Can you work these out from the model? Positions are in its coordinate system, mm. Face numbers are marked on the shaded views. A direction names the side the tool comes from. Coordinates: 2 decimals unless noted, no trailing zeros. Order: outer loops, then holes, each group sorted by start corner. A loop starts at its lowest first (then second) coordinate and runs counter-clockwise, first axis right, second up. Notation, with made-up numbers: (35, 77.5) - (92, 77.5) arc R22 ccw to (92, 115.5) - close; hole circle Ø2 at (35.5, 21). An arc over 180 degrees is marked (long way). Use a Markdown table: item, result. Add a question column.
(1) I want a section at C-C (z = 1.6). List the corners of the cut face in (x, y) for me, and give its area (3 significant figures).
(2) I want a section at D-D (y = 14). List the corners of the cut face in (x, z) for me, and give its area (3 significant figures).
(3) If I drill on L1, parallel to Y at x = 9.75, z = 1.5; L2, parallel to X at y = 9, z = 0.8; L3, parallel to X at y = 3.5, z = 2.2, over which ranges is the centre line in solid material (lowest first)? Write a range as [from, to].
(4) For pin 1 Ø0.6 at (x, z) = (11.5, 2) entering from -Y; pin 2 Ø0.8 at (x, z) = (12, 0.5) entering from -Y; pin 3 Ø5 at (x, y) = (-1, 13.5) entering from -Z; pin 4 Ø0.6 at (x, y) = (9, 17.5) entering from -Z, each with a flat end and sliding along its axis, tell me the tip position at first contact or that it passes through.
(5) On a 3-axis mill with a long thin cutter (end or side, diameter ignored), from which of +Z, -Z, +X, -X, +Y, -Y can I reach the whole of each face in a straight line? I mean the marked faces 1, 2 and 3. Say none if no direction works.
(6) I want a section at A-A (z = 0.5). List the corners of the cut face in (x, y) for me, and give its area (3 significant figures).
(7) I want a section at B-B (x = 7.5). List the corners of the cut face in (y, z) for me, and give its area (3 significant figures).
```python
from build123d import *

# Parameters (mm, degrees)
F1_DEPTH      = 2.35
F2_R          = 0.5
F3_DEPTH      = 5
F3_DEPTH_BACK = 5
F5_DEPTH      = 1.85
F6_R          = 0.35
F7_DEPTH      = 1.6


with BuildPart() as f1:
    # F0 (on Top) → F1 (new body)
    with BuildSketch(Plane.XY):
        with BuildLine():
            Line((12.5348381698, 18.1987490505), (10.8179235831, 18.1987490505))
            Line((10.8179235831, 18.1987490505), (9.1010301327, 18.1902297699))
            Line((9.1010301327, 18.1902297699), (7.1743787806, 17.653559883))
            Line((7.1743787806, 17.653559883), (3.98264217, 12.5729282876))
            ThreePointArc((3.98264217, 12.5729282876), (3.2243689245, 9.1481475257), (4.0165917388, 5.7310603752))
            Line((4.0165917388, 5.7310603752), (7.2585904547, 0.6823531817))
            Line((7.2585904547, 0.6823531817), (9.1909860265, 0.0613885547))
            Line((9.1909860265, 0.0613885547), (10.8629018068, 0.0696846546))
            Line((10.8629018068, 0.0696846546), (12.5348381698, 0.0696846546))
            Line((12.5348381698, 0.0696846546), (14.464128744, 0.7002301281))
            Line((14.464128744, 0.7002301281), (17.6810360095, 5.7649618728))
            ThreePointArc((17.6810360095, 5.7649618728), (18.4562935833, 9.1859379434), (17.6810360095, 12.606914014))
            Line((17.6810360095, 12.606914014), (14.464128744, 17.6716457586))
            Line((14.464128744, 17.6716457586), (12.5348381698, 18.1987490505))
        make_face()
    extrude(amount=F1_DEPTH)

    # F2 (on Right) → F3 (join, two sides)
    with BuildSketch(Plane.YZ) as f3_sk:
        with Locations((9.1614143501, 1.6)):
            Circle(F2_R)
    extrude(amount=F3_DEPTH)
    extrude(f3_sk.sketch, amount=-F3_DEPTH_BACK)

    # F4 (on face) → F5 (cut)
    with BuildSketch(Plane(origin=(0, 0, 0), x_dir=(1, 0, 0), z_dir=(0, 0, -1))):
        Polygon((7.2585904547, -0.6823531817), (7.0886202668, -0.9470447456), (9.2218469568, -0.2615441498), (10.8624056067, -0.2696846546), (12.5029844531, -0.2696846546), (14.6327834476, -0.9657618207), (14.464128744, -0.7002301281), (12.5348381698, -0.0696846546), (10.8629018068, -0.0696846546), (9.1909860265, -0.0613885547), align=None)
        Polygon((9.1288516348, -17.9903653589), (7.0162878227, -17.401909445), (7.1743787806, -17.653559883), (9.1010301327, -18.1902297699), (10.8179235831, -18.1987490505), (12.5348381698, -18.1987490505), (14.464128744, -17.6716457586), (14.623466438, -17.4207828614), (12.5080087317, -17.9987490505), (10.8184197833, -17.9987490505), align=None)
    extrude(amount=-F5_DEPTH, mode=Mode.SUBTRACT)

    # F6 (on face) → F7 (cut)
    with BuildSketch(Plane.XY.offset(2.35)):
        with Locations((12.7608353453, 0.9049560811)):
            Circle(F6_R)
        with Locations((13.8208036158, 17.0416355185)):
            Circle(F6_R)
    extrude(amount=-F7_DEPTH, mode=Mode.SUBTRACT)


solid = f1.part
```
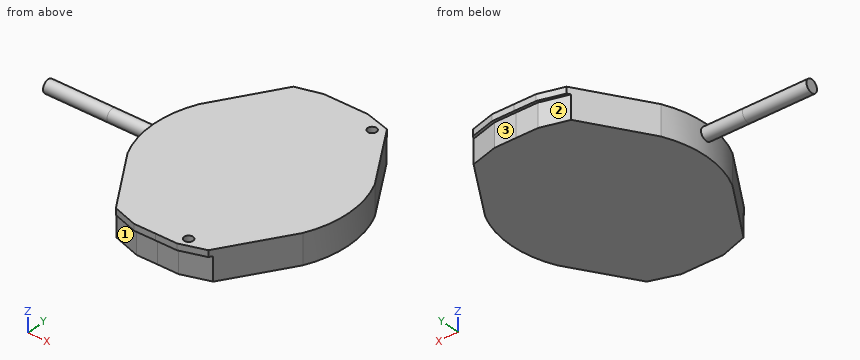
Answers follow:
| question | item | result |
|---|---|---|
| 1 | outline | (-5, 8.66) - (3.24, 8.66) arc R7.94 ccw to (4.02, 5.73) - (7.09, 0.95) - (9.22, 0.26) - (10.86, 0.27) - (12.5, 0.27) - (14.63, 0.97) - (17.68, 5.76) arc R7.94 ccw to (17.68, 12.61) - (14.62, 17.42) - (12.51, 18) - (10.82, 18) - (9.13, 17.99) - (7.02, 17.4) - (3.98, 12.57) arc R7.94 ccw to (3.24, 9.66) - (-5, 9.66) - close; hole circle Ø0.7 at (12.76, 0.9); hole circle Ø0.7 at (13.82, 17.04) |
| 1 | area | 217 mm² |
| 2 | outline | (4.88, 0) - (16.8, 0) - (16.8, 2.35) - (4.88, 2.35) - close |
| 2 | area | 28.0 mm² |
| 3 | L1 | y = [0.26, 17.99] |
| 3 | L2 | x = [3.23, 18.45] |
| 3 | L3 | x = [5.45, 16.24] |
| 4 | pin 1 | stops at y = 0.07 |
| 4 | pin 2 | stops at y = 0.27 |
| 4 | pin 3 | passes through |
| 4 | pin 4 | stops at z = 0 |
| 5 | face 1 | -Z, -X, -Y |
| 5 | face 2 | -Z, -X, +Y |
| 5 | face 3 | -Z, +X, -X, +Y |
| 6 | outline | (3.98, 12.57) arc R7.94 ccw to (4.02, 5.73) - (7.09, 0.95) - (9.22, 0.26) - (10.86, 0.27) - (12.5, 0.27) - (14.63, 0.97) - (17.68, 5.76) arc R7.94 ccw to (17.68, 12.61) - (14.62, 17.42) - (12.51, 18) - (10.82, 18) - (9.13, 17.99) - (7.02, 17.4) - close |
| 6 | area | 210 mm² |
| 7 | outline | (0.6, 1.85) - (0.81, 1.85) - (0.81, 0) - (17.54, 0) - (17.54, 1.85) - (17.74, 1.85) - (17.74, 2.35) - (0.6, 2.35) - close |
| 7 | area | 39.5 mm² |
